Verification items for the finished model (mm, model axes). A direction names the side the tool comes from. Coordinates: 2 decimals unless noted, no trailing zeros. Order: outer loops, then holes, each group sorted by start corner. A loop starts at its lowest first (then second) coordinate and runs counter-clockwise, first axis right, second up. Notation, with made-up numbers: M 72,72 L 127,72 A23 ccw 127,108 Z; hole C -2,72.25 d4. An arc over 180 degrees is marked long. Return JSON: item names as keys, results as strings. Group by question number.
1. Material ranges on line 1 along X through (y, z) = (-2.5, -39.5); line 2 along X through (y, z) = (3.5, -9.9); line 3 along Z through (x, y) = (300, -1.75), recorded low to high.
2. Mould release check, pull along Z, two halves, no side actions. Record for faces 1 (the flat face through (166, 2, 3)), 2 (the flat face through (332, 0, -32)), 3 (the flat face through (143, 8, -108)): +Z half, -Z half, draft (parallel to the pull), parting line (faces both ways), or undercut.
3. Section check B-B, the plane z = -49. Record the cut outline in (x, y), plus the area to 3 significant figures.
4. Gauge pin test, flat ends, axial feed: pin 1 (5.5 mm diameter, centred on x = 35.9, z = -9.9, fed in from -Y); pin 2 (1.8 mm diameter, centred on x = 9, z = -105.5, fed in from +Y); pin 3 (1.6 mm diameter, centred on x = 56, z = -7.5, fed in from -Y). Record the tip position at first contact, or that the pin passes through.
5. Set-up check for faces 4 (the flat face through (332.5, 4.5, -97.7)), 5 (the flat face through (12.9, 3, -10)), 6 (the flat face through (166, -2, 0)): record each of +Z, -Z, +X, -X, +Y, -Y from which the full face is reachable in a straight line by a thin tool's end or side.
6. Section check A-A, the plane x = 154. Record the cut outline in (y, z), plus the area to 3 significant figures.
```python
from build123d import *

# Parameters (mm, degrees)
SKETCH_1_W              = 337.35
SKETCH_1_H              = 116.87
SKETCH_1_W_2            = 324.05
SKETCH_1_H_2            = 103.07
EXTRUDE_1_DEPTH         = 8
FILLET_1_R              = 5
HOLE_WIZARD_3_2_3_2_1_D = 3.2
SKETCH_5_W              = 32
SKETCH_5_H              = 1.5
CUT_EXTRUDE_1_DEPTH     = 355.911853
EXTRUDE_2_REACH         = 356.912
SKETCH_6_W              = 3
SKETCH_6_H              = 8
SKETCH_7_W              = 257.05
SKETCH_7_H              = 8
EXTRUDE_3_DEPTH         = 4
SKETCH_8_W              = 257.05
SKETCH_8_H              = 4
EXTRUDE_4_DEPTH         = 3
SKETCH_11_W             = 99.07
SKETCH_11_H             = 11
EXTRUDE_5_DEPTH         = 2
SKETCH_13_W             = 42
SKETCH_13_H             = 4.5
CUT_EXTRUDE_2_DEPTH     = 354.692894189
SKETCH_14_W             = 121.5
SKETCH_14_H             = 1.5
CUT_EXTRUDE_3_DEPTH     = 355.911853
SKETCH_16_W             = 32
SKETCH_16_H             = 6.5
EXTRUDE_7_DEPTH         = 4
SKETCH_17_W             = 103.07
SKETCH_17_H             = 3
CUT_EXTRUDE_4_DEPTH     = 0.1
EXTRUDE_8_DEPTH         = 2
SKETCH_19_W             = 70.55
SKETCH_19_H             = 2
SKETCH_19_W_2           = 95
EXTRUDE_9_DEPTH         = 3
SKETCH_20_R             = 3.5
CUT_EXTRUDE_5_DEPTH     = 4
EXTRUDE_10_DEPTH        = 12
SKETCH_22_W             = 44.9064152
SKETCH_22_H             = 4
CUT_EXTRUDE_6_DEPTH     = 9.9
SKETCH_23_W             = 6
SKETCH_23_H             = 6
SKETCH_23_R             = 2.15
EXTRUDE_11_DEPTH        = 3
SKETCH_26_W             = 5.2
SKETCH_26_H             = 6
SKETCH_26_W_2           = 6
EXTRUDE_12_DEPTH        = 6
SKETCH_27_W             = 6
SKETCH_27_H             = 6
EXTRUDE_13_DEPTH        = 3
SKETCH_28_R             = 2.15
CUT_EXTRUDE_7_DEPTH     = 4.2
CUT_EXTRUDE_8_REACH     = 362.981
SKETCH_29_W             = 0.1
SKETCH_29_H             = 0.921954446
SKETCH_30_R             = 3.75
CUT_EXTRUDE_9_DEPTH     = 3.5
FILLET_3_R              = 1


with BuildPart() as part:
    # 草图1 → 凸台-拉伸1 (new body)
    with BuildSketch(Plane(origin=(0, 0, 0), x_dir=(1, 0, 0), z_dir=(0, 1, 0))):
        with Locations((168.675, 58.435)):
            Rectangle(SKETCH_1_W, SKETCH_1_H)
        with Locations((168.925, 58.435)):
            Rectangle(SKETCH_1_W_2, SKETCH_1_H_2, mode=Mode.SUBTRACT)
    extrude(amount=EXTRUDE_1_DEPTH)

    # 圆角1
    fillet_1_edges = [part.edges().sort_by_distance(p)[0] for p in [
        (0, 4, -116.87),
        (337.35, 4, -116.87),
        (337.35, 4, 0),
        (0, 4, 0),
    ]]
    fillet(fillet_1_edges, radius=FILLET_1_R)

    # Ø3.2 (3.2) 直径孔1 (through all)
    with Locations(Plane(origin=(0, 8, 0), x_dir=(1, 0, 0), z_dir=(0, 1, 0))):
        with Locations((3.45, 98.435), (87.17, 113.42), (247.17, 113.42), (334.15, 98.435), (334.15, 18.435), (247.17, 3.45), (87.17, 3.45), (3.45, 18.435)):
            Hole(HOLE_WIZARD_3_2_3_2_1_D / 2)

    # 草图5 → 切除-拉伸1 (cut, through all)
    with BuildSketch(Plane.XY.offset(-109.97)):
        with Locations((57.9, 0.75)):
            Rectangle(SKETCH_5_W, SKETCH_5_H)
    extrude(amount=-CUT_EXTRUDE_1_DEPTH, mode=Mode.SUBTRACT)

    # 草图6 → 凸台-拉伸2 (add, up to next)
    with BuildSketch(Plane.XY.offset(-109.97), mode=Mode.PRIVATE) as extrude_2_sk1:
        with Locations((40.4, 4)):
            Rectangle(SKETCH_6_W, SKETCH_6_H)
    extrude_2_tool1 = extrude(extrude_2_sk1.sketch, amount=EXTRUDE_2_REACH, mode=Mode.PRIVATE) - part.part
    add(extrude_2_tool1.solids().sort_by_distance((40.4, 4, -109.97))[0])

    # 草图7 → 凸台-拉伸3 (add)
    with BuildSketch(Plane.XY.offset(-109.97)):
        with Locations((202.425, 4)):
            Rectangle(SKETCH_7_W, SKETCH_7_H)
    extrude(amount=EXTRUDE_3_DEPTH)

    # 草图8 → 凸台-拉伸4 (add)
    with BuildSketch(Plane.XZ):
        with Locations((202.425, -107.97)):
            Rectangle(SKETCH_8_W, SKETCH_8_H)
    extrude(amount=EXTRUDE_4_DEPTH)

    # 草图11 → 凸台-拉伸5 (add)
    with BuildSketch(Plane.ZY.offset(-330.95)):
        with Locations((-56.435, 2.5)):
            Rectangle(SKETCH_11_W, SKETCH_11_H)
    extrude(amount=EXTRUDE_5_DEPTH)

    # 草图13 → 切除-拉伸2 (cut, through all)
    with BuildSketch(Plane.XY.offset(-105.97)):
        with Locations((307.95, -0.75)):
            Rectangle(SKETCH_13_W, SKETCH_13_H)
    extrude(amount=-CUT_EXTRUDE_2_DEPTH, mode=Mode.SUBTRACT)

    # 草图14 → 切除-拉伸3 (cut, through all)
    with BuildSketch(Plane(origin=(0, 0, -6.9), x_dir=(-1, 0, 0), z_dir=(0, 0, -1))):
        with Locations((-173.2, 0.75)):
            Rectangle(SKETCH_14_W, SKETCH_14_H)
    extrude(amount=-CUT_EXTRUDE_3_DEPTH, mode=Mode.SUBTRACT)

    # 草图16 → 凸台-拉伸7 (add)
    with BuildSketch(Plane.XY.offset(-109.97)):
        with Locations((57.9, 4.75)):
            Rectangle(SKETCH_16_W, SKETCH_16_H)
    extrude(amount=EXTRUDE_7_DEPTH)

    # 草图17 → 切除-拉伸4 (cut)
    with BuildSketch(Plane(origin=(330.95, 0, 0), x_dir=(0, 0, -1), z_dir=(1, 0, 0))):
        with Locations((58.435, -1.5)):
            Rectangle(SKETCH_17_W, SKETCH_17_H)
    extrude(amount=-CUT_EXTRUDE_4_DEPTH, mode=Mode.SUBTRACT)

    # 草图18 → 凸台-拉伸8 (add)
    with BuildSketch(Plane(origin=(0, 0, -6.9), x_dir=(-1, 0, 0), z_dir=(0, 0, -1))):
        Polygon((-233.95, 0), (-233.95, 1.5), (-112.45, 1.5), (-112.45, 0), (-41.9, 0), (-41.9, 8), (-328.95, 8), (-328.95, 0), align=None)
    extrude(amount=EXTRUDE_8_DEPTH)

    # 草图19 → 凸台-拉伸9 (add)
    with BuildSketch(Plane.XZ):
        with Locations((77.175, -7.9)):
            Rectangle(SKETCH_19_W, SKETCH_19_H)
        with Locations((281.45, -7.9)):
            Rectangle(SKETCH_19_W_2, SKETCH_19_H)
    extrude(amount=EXTRUDE_9_DEPTH)

    # 草图20 → 切除-拉伸5 (cut)
    with BuildSketch(Plane.XZ.offset(3)):
        with Locations((92.088456012, -9.54)):
            Circle(SKETCH_20_R)
        with Locations((262.268456012, -9.54)):
            Circle(SKETCH_20_R)
        with Locations((328.308456012, -13.35)):
            Circle(SKETCH_20_R)
        with Locations((328.308456012, -74.31)):
            Circle(SKETCH_20_R)
        with Locations((137.808456012, -107.33)):
            Circle(SKETCH_20_R)
        with Locations((22.238456012, -9.54)):
            Circle(SKETCH_20_R)
        with Locations((9.538456012, -23.51)):
            Circle(SKETCH_20_R)
        with Locations((9.538456012, -103.52)):
            Circle(SKETCH_20_R)
    extrude(amount=-CUT_EXTRUDE_5_DEPTH, mode=Mode.SUBTRACT)

    # 草图21 → 凸台-拉伸10 (add)
    with BuildSketch(Plane(origin=(0, 8, 0), x_dir=(1, 0, 0), z_dir=(0, 1, 0))):
        with BuildLine():
            Line((-3, 111.87), (-3, 5))
            ThreePointArc((-3, 5), (-0.656854249, -0.656854249), (5, -3))
            Line((5, -3), (332.35, -3))
            ThreePointArc((332.35, -3), (338.006854249, -0.656854249), (340.35, 5))
            Line((340.35, 5), (340.35, 111.87))
            ThreePointArc((340.35, 111.87), (338.006854249, 117.526854249), (332.35, 119.87))
            Line((332.35, 119.87), (5, 119.87))
            ThreePointArc((5, 119.87), (-0.656854249, 117.526854249), (-3, 111.87))
        make_face()
        with BuildLine():
            Line((0, 111.87), (0, 5))
            ThreePointArc((0, 5), (1.464466094, 1.464466094), (5, 0))
            Line((5, 0), (332.35, 0))
            ThreePointArc((332.35, 0), (335.885533906, 1.464466094), (337.35, 5))
            Line((337.35, 5), (337.35, 111.87))
            ThreePointArc((337.35, 111.87), (335.885533906, 115.405533906), (332.35, 116.87))
            Line((332.35, 116.87), (5, 116.87))
            ThreePointArc((5, 116.87), (1.464466094, 115.405533906), (0, 111.87))
        make_face(mode=Mode.SUBTRACT)
    extrude(amount=-EXTRUDE_10_DEPTH)

    # 草图22 → 切除-拉伸6 (cut)
    with BuildSketch(Plane(origin=(0, 0, -119.87), x_dir=(-1, 0, 0), z_dir=(0, 0, -1))):
        with Locations((-33.455248412, -2)):
            Rectangle(SKETCH_22_W, SKETCH_22_H)
    extrude(amount=-CUT_EXTRUDE_6_DEPTH, mode=Mode.SUBTRACT)

    # 草图23 → 凸台-拉伸11 (add)
    # profile 1 of 5: a face of its own
    with BuildSketch(Plane.XZ):
        with Locations((9.9, -9.9)):
            Rectangle(SKETCH_23_W, SKETCH_23_H)
    # profile 2 of 5: a face of its own
    with BuildSketch(Plane.XZ):
        with Locations((35.9, -9.9)):
            Rectangle(SKETCH_23_W, SKETCH_23_H)
    # profile 3 of 5: a face of its own
    with BuildSketch(Plane.XZ):
        with Locations((9.9, -106.97)):
            Rectangle(SKETCH_23_W, SKETCH_23_H)
        with Locations(Location((9.9, -106.97, 0), (0, 0, 270))):
            Circle(SKETCH_23_R, mode=Mode.SUBTRACT)
    # profile 4 of 5: a face of its own
    with BuildSketch(Plane.XZ):
        with Locations((9.9, -84.17)):
            Rectangle(SKETCH_23_W, SKETCH_23_H)
        with Locations(Location((9.9, -84.17, 0), (0, 0, 270))):
            Circle(SKETCH_23_R, mode=Mode.SUBTRACT)
    # profile 5 of 5: a face of its own
    with BuildSketch(Plane.XZ):
        with Locations((30.7, -106.97)):
            Rectangle(SKETCH_23_W, SKETCH_23_H)
        with Locations(Location((30.7, -106.97, 0), (0, 0, 270))):
            Circle(SKETCH_23_R, mode=Mode.SUBTRACT)
    extrude(amount=-EXTRUDE_11_DEPTH)

    # 草图26 → 凸台-拉伸12 (add)
    with BuildSketch(Plane.XZ):
        with Locations((36.3, -106.97)):
            Rectangle(SKETCH_26_W, SKETCH_26_H)
        with Locations((9.9, -78.17)):
            Rectangle(SKETCH_26_W_2, SKETCH_26_H)
    extrude(amount=-EXTRUDE_12_DEPTH)

    # 草图27 → 凸台-拉伸13 (add)
    with BuildSketch(Plane(origin=(0, 3, 0), x_dir=(1, 0, 0), z_dir=(0, 1, 0))):
        with Locations((9.9, 9.9)):
            Rectangle(SKETCH_27_W, SKETCH_27_H)
        with Locations((35.9, 9.9)):
            Rectangle(SKETCH_27_W, SKETCH_27_H)
    extrude(amount=EXTRUDE_13_DEPTH)

    # 草图28 → 切除-拉伸7 (cut)
    with BuildSketch(Plane(origin=(0, 6, 0), x_dir=(1, 0, 0), z_dir=(0, 1, 0))):
        with Locations(Location((35.9, 106.97, 0), (0, 0, 270))):
            Circle(SKETCH_28_R)
        with Locations(Location((35.9, 9.9, 0), (0, 0, 270))):
            Circle(SKETCH_28_R)
        with Locations(Location((9.9, 9.9, 0), (0, 0, 270))):
            Circle(SKETCH_28_R)
        with Locations(Location((9.9, 78.17, 0), (0, 0, 270))):
            Circle(SKETCH_28_R)
    extrude(amount=-CUT_EXTRUDE_7_DEPTH, mode=Mode.SUBTRACT)

    # 切除-拉伸8: up to this face of the body (flat: up to its plane)
    cut_extrude_8_end = Plane(part.part.faces().sort_by_distance((35.9, 1.8, -106.97))[0])
    # 草图29 → 切除-拉伸8 (cut, up to the picked face)
    with BuildSketch(Plane(origin=(0, 6, 0), x_dir=(1, 0, 0), z_dir=(0, 1, 0)), mode=Mode.PRIVATE) as cut_extrude_8_sk1:
        with Locations((33.75, 106.97)):
            Rectangle(SKETCH_29_W, SKETCH_29_H)
    cut_extrude_8_tool1 = split(extrude(cut_extrude_8_sk1.sketch, amount=-CUT_EXTRUDE_8_REACH, mode=Mode.PRIVATE), bisect_by=cut_extrude_8_end, keep=Keep.BOTH, mode=Mode.PRIVATE)
    add(cut_extrude_8_tool1.solids().sort_by(Axis((33.75, 6, -106.97), (0, -1, 0)))[0], mode=Mode.SUBTRACT)

    # 草图30 → 切除-拉伸9 (cut)
    with BuildSketch(Plane(origin=(0, 8, 0), x_dir=(1, 0, 0), z_dir=(0, 1, 0))):
        with Locations(Location((87.17, 113.42, 0), (0, 0, 270))):
            Circle(SKETCH_30_R)
        with Locations(Location((247.17, 113.42, 0), (0, 0, 270))):
            Circle(SKETCH_30_R)
        with Locations(Location((334.15, 98.435, 0), (0, 0, 270))):
            Circle(SKETCH_30_R)
        with Locations(Location((334.15, 18.435, 0), (0, 0, 270))):
            Circle(SKETCH_30_R)
        with Locations(Location((87.17, 3.45, 0), (0, 0, 270))):
            Circle(SKETCH_30_R)
        with Locations(Location((247.17, 3.45, 0), (0, 0, 270))):
            Circle(SKETCH_30_R)
        with Locations((3.45, 18.435)):
            Circle(SKETCH_30_R)
        with Locations((3.45, 98.435)):
            Circle(SKETCH_30_R)
    extrude(amount=-CUT_EXTRUDE_9_DEPTH, mode=Mode.SUBTRACT)

    # 圆角3
    fillet_3_edges = [part.edges().sort_by_distance(p)[0] for p in [
        (-0.656854249, 8, -117.526854249),
        (-3, 8, -58.435),
        (-0.656854249, 8, 0.656854249),
        (168.675, 8, 3),
        (338.006854249, 8, 0.656854249),
        (340.35, 8, -58.435),
        (338.006854249, 8, -117.526854249),
        (168.675, 8, -119.87),
    ]]
    fillet(fillet_3_edges, radius=FILLET_3_R)


solid = part.part
```
Answers follow:
{
 "1": {"line 1": "-3 to 0, 328.95 to 330.85, 337.35 to 340.35", "line 2": "-3 to 7.75, 12.05 to 12.9, 32.9 to 33.75, 38.05 to 41.9, 328.95 to 340.35", "line 3": "-119.87 to -116.87, -8.9 to -6.9, 0 to 3"},
 "2": {"face 1": "+Z half", "face 2": "undercut", "face 3": "draft"},
 "3": {"outline": "M -3,-4 L 0,-4 L 0,0 L 6.9,0 L 6.9,8 L -2,8 A1 ccw -3,7 Z; M 38.9,0 L 41.9,0 L 41.9,8 L 38.9,8 Z; M 328.95,-3 L 330.85,-3 L 330.85,0 L 337.35,0 L 337.35,-4 L 340.35,-4 L 340.35,7 A1 ccw 339.35,8 L 328.95,8 Z", "area": "224 mm^2"},
 "4": {"pin 1": "y = 0", "pin 2": "y = 3", "pin 3": "y = -3"},
 "5": {"face 4": "+Y", "face 5": "+Y, -Y", "face 6": "-Y"},
 "6": {"outline": "M -4,-119.87 L 7,-119.87 A1 ccw 8,-118.87 L 8,-105.97 L -3,-105.97 L -3,-109.97 L 0,-109.97 L 0,-116.87 L -4,-116.87 Z; M -4,0 L 1.5,0 L 1.5,-8.9 L 8,-8.9 L 8,2 A1 ccw 7,3 L -4,3 Z", "area": "229 mm^2"}
}
